Here's how the part is built. I have some questions about the finished solid (model axes, mm). Face numbers are marked on the shaded views. A direction names the side the tool comes from. Coordinates: 2 decimals unless noted, no trailing zeros. Write each loop counter-clockwise with the first axis right and the second up, starting at its lowest first coordinate (ties: lowest second). Pieces come first, ordered by that corner, then holes.
Item 1: For the marked faces 4, 5 and 6, which set-ups out of +Z, -Z, +X, -X, +Y, -Y let a thin tool reach every point of the face, with its end or its side?
Item 2: Please list where these lines run through material, in increasing order: line 1 (Z direction, x = 5.75, y = -0.25); line 2 (X direction, y = 4.25, z = -4.25); line 3 (Y direction, x = -5, z = -0.75).
Item 3: If we mould it in two halves opening along Z, with no side actions, what happens to the marked faces 1, 2 and 3? For each: pulls with the +Z half, pulls with the -Z half, needs draft (parallel to the pull), parting line crosses it, or undercut.
Item 4: I'm going to push flat-ended pins straight in: P1, Ø0.6, axis at x = 5, z = -1, coming from the +Y side; P2, Ø2, axis at x = -6, z = -5.5, coming from the -Y side; P3, Ø6, axis at x = 5, y = 5, coming from the -Z side; P4, Ø2.5, axis at y = 4.5, z = 1, coming from the -X side. Where does each tip first touch, or does it pass through?
Item 5: I want a section at D-D (x = -0.5). Please give me the cut outline in (y, z).
Item 6: I want a section at B-B (y = -3.75). Count the separate pieces of the cut face and the enclosed holes in it, and give its area (3 significant figures).
Item 7: I want a section at C-C (z = -1). Please give me the cut outline in (x, y), and give its area (3 significant figures).
Item 8: I want a section at A-A (y = 4). Please give me the cut outline in (x, z).
from build123d import *

# Parameters (mm, degrees)
SKETCH1_W               = 20.3
SKETCH1_H               = 15.2
BOSS_EXTRUDE1_DEPTH     = 1.56
SKETCH2_W               = 20.3
SKETCH2_H               = 2.4
BOSS_EXTRUDE2_DEPTH     = 2.52
SKETCH3_R               = 0.2
BOSS_EXTRUDE3_DEPTH     = 3.2
LPATTERN1_COUNT         = 8
LPATTERN1_PITCH         = 2.54
MIRROR1_COPY_1_SKETCH_R = 0.2
MIRROR1_COPY_1_DEPTH    = 3.2
MIRROR1_COPY_2_SKETCH_R = 0.2
MIRROR1_COPY_2_DEPTH    = 3.2
MIRROR1_COPY_3_SKETCH_R = 0.2
MIRROR1_COPY_3_DEPTH    = 3.2
MIRROR1_COPY_4_SKETCH_R = 0.2
MIRROR1_COPY_4_DEPTH    = 3.2
MIRROR1_COPY_5_SKETCH_R = 0.2
MIRROR1_COPY_5_DEPTH    = 3.2
MIRROR1_COPY_6_SKETCH_R = 0.2
MIRROR1_COPY_6_DEPTH    = 3.2
MIRROR1_COPY_7_SKETCH_R = 0.2
MIRROR1_COPY_7_DEPTH    = 3.2
SKETCH4_W               = 5.3
SKETCH4_H               = 8.8
BOSS_EXTRUDE4_DEPTH     = 5.3
SKETCH5_W               = 1.1
SKETCH5_H               = 3.5
CUT_EXTRUDE1_DEPTH      = 5.3


with BuildPart() as part:
    # Sketch1 → Boss-Extrude1 (new body)
    with BuildSketch(Plane(origin=(0, 0, 0), x_dir=(1, 0, 0), z_dir=(0, 1, 0))):
        Rectangle(SKETCH1_W, SKETCH1_H)
    extrude(amount=BOSS_EXTRUDE1_DEPTH)

    # Sketch2 → Boss-Extrude2 (add)
    with BuildSketch(Plane.XZ):
        with Locations((0, 6.4)):
            Rectangle(SKETCH2_W, SKETCH2_H)
        with Locations((0, -6.4)):
            Rectangle(SKETCH2_W, SKETCH2_H)
    extrude(amount=BOSS_EXTRUDE2_DEPTH)

    # Sketch3 → Boss-Extrude3 (add)
    with BuildSketch(Plane.XZ.offset(2.52)):
        with Locations((-8.89, 6.35)):
            Circle(SKETCH3_R)
    boss_extrude3 = extrude(amount=BOSS_EXTRUDE3_DEPTH)

    # LPattern1: Boss-Extrude3 ×8
    with Locations(*[(i * LPATTERN1_PITCH, 0, 0) for i in range(1, LPATTERN1_COUNT)]):
        add(boss_extrude3)

    # Mirror1: Boss-Extrude3 across plane
    add(boss_extrude3.mirror(Plane.XY))

    # Mirror1 copy 1 sketch → Mirror1 copy 1 (add)
    with BuildSketch(Plane(origin=(2.54, -2.52, 0), x_dir=(1, 0, 0), z_dir=(0, -1, 0))):
        with Locations((-8.89, -6.35)):
            Circle(MIRROR1_COPY_1_SKETCH_R)
    extrude(amount=MIRROR1_COPY_1_DEPTH)

    # Mirror1 copy 2 sketch → Mirror1 copy 2 (add)
    with BuildSketch(Plane(origin=(5.08, -2.52, 0), x_dir=(1, 0, 0), z_dir=(0, -1, 0))):
        with Locations((-8.89, -6.35)):
            Circle(MIRROR1_COPY_2_SKETCH_R)
    extrude(amount=MIRROR1_COPY_2_DEPTH)

    # Mirror1 copy 3 sketch → Mirror1 copy 3 (add)
    with BuildSketch(Plane(origin=(7.62, -2.52, 0), x_dir=(1, 0, 0), z_dir=(0, -1, 0))):
        with Locations((-8.89, -6.35)):
            Circle(MIRROR1_COPY_3_SKETCH_R)
    extrude(amount=MIRROR1_COPY_3_DEPTH)

    # Mirror1 copy 4 sketch → Mirror1 copy 4 (add)
    with BuildSketch(Plane(origin=(10.16, -2.52, 0), x_dir=(1, 0, 0), z_dir=(0, -1, 0))):
        with Locations((-8.89, -6.35)):
            Circle(MIRROR1_COPY_4_SKETCH_R)
    extrude(amount=MIRROR1_COPY_4_DEPTH)

    # Mirror1 copy 5 sketch → Mirror1 copy 5 (add)
    with BuildSketch(Plane(origin=(12.7, -2.52, 0), x_dir=(1, 0, 0), z_dir=(0, -1, 0))):
        with Locations((-8.89, -6.35)):
            Circle(MIRROR1_COPY_5_SKETCH_R)
    extrude(amount=MIRROR1_COPY_5_DEPTH)

    # Mirror1 copy 6 sketch → Mirror1 copy 6 (add)
    with BuildSketch(Plane(origin=(15.24, -2.52, 0), x_dir=(1, 0, 0), z_dir=(0, -1, 0))):
        with Locations((-8.89, -6.35)):
            Circle(MIRROR1_COPY_6_SKETCH_R)
    extrude(amount=MIRROR1_COPY_6_DEPTH)

    # Mirror1 copy 7 sketch → Mirror1 copy 7 (add)
    with BuildSketch(Plane(origin=(17.78, -2.52, 0), x_dir=(1, 0, 0), z_dir=(0, -1, 0))):
        with Locations((-8.89, -6.35)):
            Circle(MIRROR1_COPY_7_SKETCH_R)
    extrude(amount=MIRROR1_COPY_7_DEPTH)

    # Sketch4 → Boss-Extrude4 (add)
    with BuildSketch(Plane(origin=(0, 1.56, 0), x_dir=(1, 0, 0), z_dir=(0, 1, 0))):
        with Locations((4.4, 0)):
            Rectangle(SKETCH4_W, SKETCH4_H)
    extrude(amount=BOSS_EXTRUDE4_DEPTH)

    # Sketch5 → Cut-Extrude1 (cut)
    with BuildSketch(Plane(origin=(7.05, 0, 0), x_dir=(0, 0, -1), z_dir=(1, 0, 0))):
        with Locations((-3.3, 5.11)):
            Rectangle(SKETCH5_W, SKETCH5_H)
        with Locations((-1.1, 5.11)):
            Rectangle(SKETCH5_W, SKETCH5_H)
        with Locations((1.1, 5.11)):
            Rectangle(SKETCH5_W, SKETCH5_H)
        with Locations((3.3, 5.11)):
            Rectangle(SKETCH5_W, SKETCH5_H)
    extrude(amount=-CUT_EXTRUDE1_DEPTH, mode=Mode.SUBTRACT)


solid = part.part
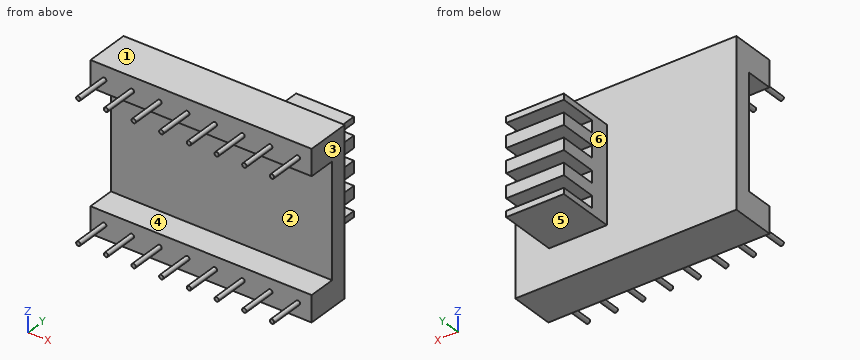
Answer:
1. face 4: +X, -X, -Y
1. face 5: -Z, +X, -X, +Y
1. face 6: +Z, -Z, -X, +Y
2. line 1: z = -7.6 to -5.2, 5.2 to 7.6
2. line 2: x = 1.75 to 7.05
2. line 3: y = 0 to 1.56
3. face 1: pulls with the +Z half
3. face 2: undercut
3. face 3: needs draft
4. P1: stops at y = 3.36
4. P2: stops at y = -5.72
4. P3: stops at z = -4.4
4. P4: stops at x = 1.75
5. outline: (-2.52, -7.6) - (1.56, -7.6) - (1.56, 7.6) - (-2.52, 7.6) - (-2.52, 5.2) - (0, 5.2) - (0, -5.2) - (-2.52, -5.2) - close
6. separate pieces: 16
6. enclosed holes: 0
6. area: 2.01 mm2
7. outline: (-10.15, 0) - (10.15, 0) - (10.15, 1.56) - (7.05, 1.56) - (7.05, 3.36) - (1.75, 3.36) - (1.75, 1.56) - (-10.15, 1.56) - close
7. area: 41.2 mm2
8. outline: (1.75, -4.4) - (7.05, -4.4) - (7.05, -3.85) - (1.75, -3.85) - close; (1.75, -2.75) - (7.05, -2.75) - (7.05, -1.65) - (1.75, -1.65) - close; (1.75, -0.55) - (7.05, -0.55) - (7.05, 0.55) - (1.75, 0.55) - close; (1.75, 1.65) - (7.05, 1.65) - (7.05, 2.75) - (1.75, 2.75) - close; (1.75, 3.85) - (7.05, 3.85) - (7.05, 4.4) - (1.75, 4.4) - close
